Input: part model. Units: mm. Frame: model coordinates. Face numbers are marked on the shaded views. A direction names the side the tool comes from. Round coordinates to 2 decimals unless told otherwise and drop trailing zeros. Loops run counter-clockwise (first coordinate to the right, second up) from the corner with the lowest first, then second, coordinate; pieces in that order, holes last. Notation, with made-up numbers: (-14.75, 31) -> (28.25, 31) arc R32 cw to (28.25, 65) -> close; hole circle Ø10 at (-23.75, 42.5). An arc over 180 degrees is marked (long way). Answer as a JSON object with one key per item and string values. Group by question number.
Item 1: Section query C-C on x = 7. Return loops of the section in (y, z).
Item 2: Section query A-A on x = -8.5. Return loops of the section in (y, z).
Item 3: Set-up query: the marked faces 1, 2 and 3. Return all of +Z, -Z, +X, -X, +Y, -Y with unobstructed straight access to the full face (end or side cutting, diameter ignored); none if empty.
Item 4: Section query B-B on y = 1.4. Return loops of the section in (x, z), and give its area (3 significant figures).
Item 5: Draft query along X for the marked faces 4, 5 and 6. Return one class per face: released by +X, released by -X, zero draft, split by the parting line, or undercut.
Item 6: Pin query (flat end, axial travel): pin 1 (2 mm diameter, centred on x = 1.5, y = 0.5, fed in from -Z). Return the tip coordinate at first contact, or that it passes through.
Item 7: Material intervals for line 1 (X direction, y = 3.3, z = 0); line 2 (X direction, y = 3.5, z = 1); line 3 (X direction, y = 3.85, z = 2.25), sorted ascending. Write a range as [from, to].
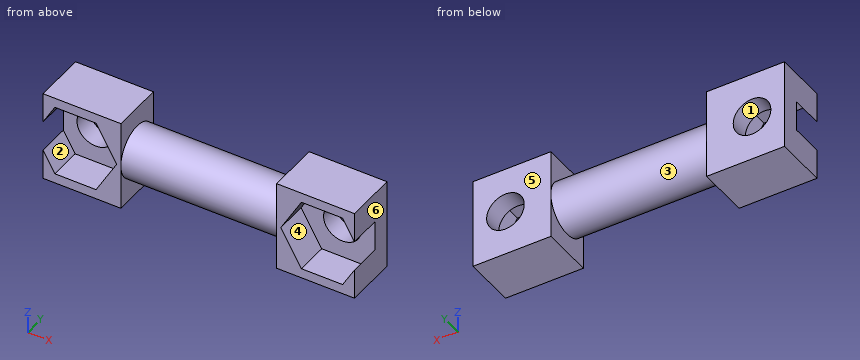
from build123d import *

# Parameters (mm, degrees)
SKETCH_1_W          = 24
SKETCH_1_H          = 7
SKETCH_1_R          = 1.45
EXTRUDE_1_DEPTH     = 4
CUT_EXTRUDE_1_DEPTH = 2.5
SKETCH_3_W          = 8.18570746
SKETCH_3_H          = 5.156071163
SKETCH_3_R          = 2
CUT_EXTRUDE_2_DEPTH = 6


with BuildPart() as part:
    # Эскиз1 → Бобышка-Вытянуть1 (new body)
    with BuildSketch(Plane(origin=(0, 0, 0), x_dir=(1, 0, 0), z_dir=(0, 1, 0))):
        Rectangle(SKETCH_1_W, SKETCH_1_H)
        with Locations(Location((-9.5, 0, 0), (0, 0, 270))):
            Circle(SKETCH_1_R, mode=Mode.SUBTRACT)
        with Locations(Location((9.5, 0, 0), (0, 0, 270))):
            Circle(SKETCH_1_R, mode=Mode.SUBTRACT)
    extrude(amount=EXTRUDE_1_DEPTH)

    # Эскиз2 → Вырез-Вытянуть1 (cut)
    with BuildSketch(Plane.XZ):
        Polygon((-7.91228676, 2.75), (-11.08771324, 2.75), (-12.675426481, 0), (-11.08771324, -2.75), (-7.91228676, -2.75), (-6.324573519, 0), align=None)
        Polygon((7.91228676, -2.75), (11.08771324, -2.75), (12.675426481, 0), (11.08771324, 2.75), (7.91228676, 2.75), (6.324573519, 0), align=None)
    extrude(amount=-CUT_EXTRUDE_1_DEPTH, mode=Mode.SUBTRACT)

    # Эскиз3 → Вырез-Вытянуть2 (cut, symmetric)
    with BuildSketch(Plane(origin=(0, 0, 0), x_dir=(0, 0, -1), z_dir=(1, 0, 0))):
        with Locations((0.188463291, 1.886210844)):
            Rectangle(SKETCH_3_W, SKETCH_3_H)
        with Locations(Location((0, 2, 0), (0, 0, 90))):
            Circle(SKETCH_3_R, mode=Mode.SUBTRACT)
    extrude(amount=CUT_EXTRUDE_2_DEPTH, both=True, mode=Mode.SUBTRACT)


solid = part.part
Solved:
{
 "1": {"outline": "(0, -3.5) -> (4, -3.5) -> (4, 3.5) -> (0, 3.5) -> (0, 1.17) -> (2.5, 1.17) -> (2.5, -1.17) -> (0, -1.17) -> close"},
 "2": {"outline": "(0, -3.5) -> (4, -3.5) -> (4, -1.05) -> (2.5, -1.05) -> (2.5, -2.75) -> (0, -2.75) -> close; (0, 2.75) -> (2.5, 2.75) -> (2.5, 1.05) -> (4, 1.05) -> (4, 3.5) -> (0, 3.5) -> close"},
 "3": {"face 1": "+Y, -Y", "face 2": "-Y", "face 3": "none"},
 "4": {"outline": "(-12, -3.5) -> (-6, -3.5) -> (-6, -1.91) -> (6, -1.91) -> (6, -3.5) -> (12, -3.5) -> (12, -1.17) -> (11.09, -2.75) -> (7.91, -2.75) -> (6.32, 0) -> (7.91, 2.75) -> (11.09, 2.75) -> (12, 1.17) -> (12, 3.5) -> (6, 3.5) -> (6, 1.91) -> (-6, 1.91) -> (-6, 3.5) -> (-12, 3.5) -> (-12, 1.17) -> (-11.09, 2.75) -> (-7.91, 2.75) -> (-6.32, 0) -> (-7.91, -2.75) -> (-11.09, -2.75) -> (-12, -1.17) -> close", "area": "79.0 mm²"},
 "5": {"face 4": "undercut", "face 5": "zero draft", "face 6": "released by +X"},
 "6": {"pin 1": "z = -1.94"},
 "7": {"line 1": "[-12, -10.95], [-8.05, 8.05], [10.95, 12]", "line 2": "[-12, -10.55], [-8.45, 8.45], [10.55, 12]", "line 3": "[-12, -6], [6, 12]"}
}
